Check sheet for the modelled part. Datum: model origin and axes. Units: mm. Give positions to 0.01 mm unless a question says otherwise; leave off trailing zeros. Write each loop counter-clockwise with the first axis right and the second up, starting at its lowest first coordinate (ties: lowest second). Pieces come first, ordered by that corner, then holes. Notation, with made-up numbers: (69.5, 64.5) -> (108.5, 64.5) arc R35 ccw to (108.5, 98.5) -> close; hole circle Ø6 at (-5.75, -19.5). An arc over 180 degrees is marked (long way). Use a Markdown table: item, result. Add a question column.
1. Scan lines: probe 1 along X at (y, z) = (394.75, 0); probe 2 along Y at (x, z) = (2, -1); probe 3 along Z at (x, y) = (0.25, 108). Record each from-to range of solid material in increasing order. Write a range as [from, to].
2. Cross-section at A-A (z = 0). Enter the section's corners in (x, y).
3. Gauge pin test, flat ends, axial feed: P1, Ø1.5, axis at x = 1.5, y = 191, coming from the +Z side; P2, Ø6, axis at x = -4, y = 238.5, coming from the +Z side; P3, Ø3, axis at x = 4.5, y = 248.5, coming from the +Z side. Record the tip position at first contact, or that the pin passes through.
4. Cross-section at C-C (y = 302.5). Enter the section's corners in (x, z), then the cut area to 3 significant figures.
5. Cross-section at B-B (x = 0). Enter the section's corners in (y, z), then the cut area to 3 significant figures.
from build123d import *

# Parameters (mm, degrees)
SKETCH_1_R          = 7.5
EXTRUDE_1_DEPTH     = 400
SKETCH_2_R          = 3
CUT_EXTRUDE_1_DEPTH = 20
CUT_EXTRUDE_START   = -20
SKETCH_3_R          = 3
CUT_EXTRUDE_2_DEPTH = 20


with BuildPart() as part:
    # 草图1 → 凸台-拉伸1 (new body)
    with BuildSketch(Plane(origin=(0, 0, 0), x_dir=(1, 0, 0), z_dir=(0, 1, 0))):
        with Locations(Location((0, 0, 0), (0, 0, 270))):
            Circle(SKETCH_1_R)
    extrude(amount=EXTRUDE_1_DEPTH)

    # 草图2 → 切除-拉伸1 (cut)
    with BuildSketch(Plane(origin=(0, 400, 0), x_dir=(1, 0, 0), z_dir=(0, 1, 0))):
        with Locations(Location((0, 0, 0), (0, 0, 270))):
            Circle(SKETCH_2_R)
    extrude(amount=-CUT_EXTRUDE_1_DEPTH, mode=Mode.SUBTRACT)

    # 草图3 → 切除-拉伸2 (cut)
    with BuildSketch(Plane(origin=(0, 0, 0), x_dir=(-1, 0, 0), z_dir=(0, -1, 0)).offset(CUT_EXTRUDE_START)):
        with Locations(Location((0, 0, 0), (0, 0, 270))):
            Circle(SKETCH_3_R)
    extrude(amount=CUT_EXTRUDE_2_DEPTH, mode=Mode.SUBTRACT)


solid = part.part
Worked answers:
| question | item | result |
|---|---|---|
| 1 | probe 1 | x = [-7.5, -3], [3, 7.5] |
| 1 | probe 2 | y = [20, 380] |
| 1 | probe 3 | z = [-7.5, 7.5] |
| 2 | outline | (-7.5, 0) -> (-3, 0) -> (-3, 20) -> (3, 20) -> (3, 0) -> (7.5, 0) -> (7.5, 400) -> (3, 400) -> (3, 380) -> (-3, 380) -> (-3, 400) -> (-7.5, 400) -> close |
| 3 | P1 | stops at z = 7.46 |
| 3 | P2 | stops at z = 7.43 |
| 3 | P3 | stops at z = 6.87 |
| 4 | outline | circle Ø15 at (0, 0) |
| 4 | area | 177 mm² |
| 5 | outline | (0, -7.5) -> (400, -7.5) -> (400, -3) -> (380, -3) -> (380, 3) -> (400, 3) -> (400, 7.5) -> (0, 7.5) -> (0, 3) -> (20, 3) -> (20, -3) -> (0, -3) -> close |
| 5 | area | 5,760 mm² |
